```python
from build123d import *

# Parameters (mm, degrees)
BOSS_EXTRUDE1_DEPTH = 7.112
SKETCH2_R           = 4.572
BOSS_EXTRUDE2_DEPTH = 11.176
SKETCH4_R           = 4.0005
CUT_EXTRUDE1_DEPTH  = 4.7625
SKETCH5_R           = 2.0955
CUT_EXTRUDE2_DEPTH  = 22.336


with BuildPart() as part:
    # Sketch1 → Boss-Extrude1 (new body)
    with BuildSketch(Plane(origin=(0, 0, 0), x_dir=(1, 0, 0), z_dir=(0, 1, 0))):
        Polygon((7.332348419, 0), (3.666174209, 6.35), (-3.666174209, 6.35), (-7.332348419, 0), (-3.666174209, -6.35), (3.666174209, -6.35), align=None)
    extrude(amount=BOSS_EXTRUDE1_DEPTH)

    # Sketch2 → Boss-Extrude2 (add)
    with BuildSketch(Plane(origin=(0, 7.112, 0), x_dir=(1, 0, 0), z_dir=(0, 1, 0))):
        Circle(SKETCH2_R)
    extrude(amount=BOSS_EXTRUDE2_DEPTH)

    # Sketch3 → Revolve1 (revolve)
    with BuildSketch(Plane.XY):
        Polygon((0, 18.288), (-4.572, 18.288), (-2.275167255, 21.336), (0, 21.336), align=None)
    revolve(axis=Axis((0, 24.854353551, 0), (0, -1, 0)))

    # Sketch4 → Cut-Extrude1 (cut)
    with BuildSketch(Plane.XZ):
        Circle(SKETCH4_R)
    extrude(amount=-CUT_EXTRUDE1_DEPTH, mode=Mode.SUBTRACT)

    # Sketch5 → Cut-Extrude2 (cut, through all)
    with BuildSketch(Plane(origin=(0, 21.336, 0), x_dir=(1, 0, 0), z_dir=(0, 1, 0))):
        Circle(SKETCH5_R)
    extrude(amount=-CUT_EXTRUDE2_DEPTH, mode=Mode.SUBTRACT)

    # Sketch7 → Revolve2 (revolve)
    with BuildSketch(Plane.XY):
        Polygon((-4.572, 9.398), (-5.55625, 9.966257002), (-5.55625, 15.433742998), (-4.572, 16.002), align=None)
    revolve(axis=Axis((0, 22.381556864, 0), (0, -1, 0)))


solid = part.part
```
Check sheet for the modelled part. Datum: model origin and axes. Units: mm. A direction names the side the tool comes from. Round coordinates to 2 decimals unless told otherwise and drop trailing zeros. Loops run counter-clockwise (first coordinate to the right, second up) from the corner with the lowest first, then second, coordinate; pieces in that order, holes last. Notation, with made-up numbers: (83.5, 3) - (127.5, 3) arc R30 ccw to (127.5, 40) - close; hole circle Ø1 at (86.5, 78.25). An arc over 180 degrees is marked (long way). Write item = value, one per line. Start each with the question number.
Q1. Section check D-D (x = -6). Record the boundary of the cut face in (y, z).
Q2. Section check A-A (x = 0). Record the boundary of the cut face in (y, z).
Q3. Access from +Z, -Z, +X, -X, +Y, -Y to the whole of each face (thin tool, end or side, straight path). Record for faces 1 (the face through (0, 4, 6.35)), 2 (the face through (2, 4.762, -2)), 3 (the face through (-5.3, 12.74, -1.67)), 4 (the face through (-0.991, 8.239, 4.463)).
Q4. Section check B-B (y = 6). Record the boundary of the cut face in (x, z).
Q5. Release check for a two-part mould opening along Z. For faces 5 (the face through (2, 13.17, -0.63)), 6 (the face through (5.474, 3.506, 3.219)), 7 (the face through (5, 7.112, 0)) record: pulls with the +Z half, pulls with the -Z half, needs draft (parallel to the pull), parting line crosses it, or undercut.
Q6. Thickness scan on L1, parallel to Z at x = 0, y = 2.3; L2, parallel to X at y = 17.5, z = 0; L3, parallel to Y at x = 4.75, z = -3.25. Record the ranges inside material, lowest first.
Q7. Section check C-C (y = 14.5). Record the boundary of the cut face in (x, z).
Q8. Depth check by flat-ended pin: P1, Ø4, axis at y = 12, z = -0.5, coming from the -X side; P2, Ø5, axis at x = 0, z = 0, coming from the -Y side; P3, Ø3, axis at x = 0.5, y = 14, coming from the -Z side. Enter the tip coordinate at first touch or a pass-through.
Derived:
q1.outline = (0, -2.31) - (7.11, -2.31) - (7.11, 2.31) - (0, 2.31) - close
q2.outline = (0, -6.35) - (7.11, -6.35) - (7.11, -4.57) - (9.4, -4.57) - (9.97, -5.56) - (15.43, -5.56) - (16, -4.57) - (18.29, -4.57) - (21.34, -2.28) - (21.34, -2.1) - (4.76, -2.1) - (4.76, -4) - (0, -4) - close; (0, 4) - (4.76, 4) - (4.76, 2.1) - (21.34, 2.1) - (21.34, 2.28) - (18.29, 4.57) - (16, 4.57) - (15.43, 5.56) - (9.97, 5.56) - (9.4, 4.57) - (7.11, 4.57) - (7.11, 6.35) - (0, 6.35) - close
q3.face_1 = +Z, +X, -X, +Y, -Y
q3.face_2 = -Y
q3.face_3 = +Y
q3.face_4 = none
q4.outline = (-7.33, 0) - (-3.67, -6.35) - (3.67, -6.35) - (7.33, 0) - (3.67, 6.35) - (-3.67, 6.35) - close; hole circle Ø4.19 at (0, 0)
q5.face_5 = undercut
q5.face_6 = pulls with the +Z half
q5.face_7 = needs draft
q6.L1 = -6.35 to -4, 4 to 6.35
q6.L2 = -4.57 to -2.1, 2.1 to 4.57
q6.L3 = 0 to 7.11
q7.outline = circle Ø11.11 at (0, 0); hole circle Ø4.19 at (0, 0)
q8.P1 = -5.56
q8.P2 = 4.76
q8.P3 = -5.56
